Work out the finished part from the listing and answer in its coordinate system (mm). Face numbers are marked on the shaded views. A direction names the side the tool comes from. Give positions to 0.01 mm unless a question says otherwise; leave off trailing zeros. Write each loop counter-clockwise with the first axis right and the second up, starting at its lowest first coordinate (ties: lowest second). Pieces come first, ordered by that corner, then holes.
1) Determine the mould class of the marked faces 1, 2 and 3 for opening direction Z: pulls with the +Z half, pulls with the -Z half, needs draft (parallel to the pull), parting line crosses it, or undercut.
2) Straight lines are drawn through the part: probe 1 along X at (y, z) = (2.35, -15.5); probe 2 along X at (y, z) = (0.75, -1). For each, find the intervals that lie inside material, in ascending order.
3) Find section B-B (y = 3.4). Count the separate pieces of the cut face and the enclosed holes in it, plus the area to 3 significant figures.
4) Given pin 1 Ø3 at (x, z) = (9, 21) entering from +Y; pin 2 Ø4 at (x, z) = (10.5, 16) entering from +Y, each flat-ended and moving along its own axis, determine where each tip first touches the part or whether it passes through.
5) Find section A-A (z = 26). Determine the outline of the cut face in (x, y).
6) A tool of negligible diameter and unlimited length cuts with its end or side. For the marked faces 4 and 5, from which of +Z, -Z, +X, -X, +Y, -Y can it reach the whole face along a straight path? Write none if from no direction.
Autodesk Fusion 360 part; units mm, degrees
sketch "Sketch1" plane through (0, 0, 0) normal (0, 1, 0) x (1, 0, 0)
  line L0 (35, 35) -> (-35, 35)
  line L1 (-35, 35) -> (-35, -35)
  line L2 (-35, -35) -> (35, -35)
  line L3 (35, -35) -> (35, 35)
  line L4 (35, 35) -> (-35, -35) construction
  line L5 (-35, 35) -> (35, -35) construction
  line L6 (0, 0) -> (9.2688, 9.2688) construction
  line L7 (0, 0) -> (84.8528, 84.8528) construction
  line L8 (0, 0) -> (0, 35) construction
  line L9 (12.5, 35) -> (-12.5, 35)
  line L10 (-35, 12.5) -> (-35, -12.5)
  line L11 (-12.5, -35) -> (12.5, -35)
  line L12 (35, -12.5) -> (35, 12.5)
  line L13 (20.5061, 33.234) -> (33.234, 20.5061) construction
  line L14 (23.3345, 36.0624) -> (36.0624, 23.3345)
  line L15 (12.5, 35) -> (23.3345, 36.0624)
  line L16 (35, 12.5) -> (36.0624, 23.3345)
  circle A0 centre (22.6274, 31.1127) radius 1.6
  circle A1 centre (31.1127, 22.6274) radius 1.6
  line L17 (-35, 12.5) -> (-36.0624, 23.3345)
  line L18 (-36.0624, 23.3345) -> (-23.3345, 36.0624)
  line L19 (-12.5, 35) -> (-23.3345, 36.0624)
  circle A2 centre (-22.6274, 31.1127) radius 1.6
  circle A3 centre (-31.1127, 22.6274) radius 1.6
  line L20 (-12.5, -35) -> (-23.3345, -36.0624)
  line L21 (-23.3345, -36.0624) -> (-36.0624, -23.3345)
  line L22 (-35, -12.5) -> (-36.0624, -23.3345)
  circle A4 centre (-31.1127, -22.6274) radius 1.6
  circle A5 centre (-22.6274, -31.1127) radius 1.6
  line L23 (35, -12.5) -> (36.0624, -23.3345)
  line L24 (36.0624, -23.3345) -> (23.3345, -36.0624)
  line L25 (12.5, -35) -> (23.3345, -36.0624)
  circle A6 centre (22.6274, -31.1127) radius 1.6
  circle A7 centre (31.1127, -22.6274) radius 1.6
  dimension "d3" = 70
  dimension "d4" = 70
  dimension "d5" = 120
  dimension "d6" = 25
  dimension "d7" = 12.5
  dimension "d9" = 360
  dimension "d12" = 82
  dimension "d13" = 9
  dimension "d15" = 4
  dimension "d16" = 3.2
  dimension "d17" = 6
  dimension "d18" = 6
  dimension "d20" = 360
extrude "Extrude1" add sketch "Sketch1" along normal blind 4 contours L0 L1 L2 L3 L9 L10 L11 L12 L14 L18 L21 L24
sketch "Sketch2" plane through (0, 4, 0) normal (0, 1, 0) x (-1, 0, 0)
  circle A0 centre (-22.6274, 31.1127) radius 1.6
  circle A1 centre (-31.1127, 22.6274) radius 1.6
  circle A2 centre (31.1127, -22.6274) radius 1.6
  circle A3 centre (31.1127, 22.6274) radius 1.6
  circle A4 centre (22.6274, 31.1127) radius 1.6
  circle A5 centre (22.6274, -31.1127) radius 1.6
  circle A6 centre (-31.1127, -22.6274) radius 1.6
  circle A7 centre (-22.6274, -31.1127) radius 1.6
  line L0 (24.397, 35) -> (-24.397, 35)
  line L1 (-24.397, 35) -> (-35, 24.397)
  line L2 (-35, 24.397) -> (-35, -24.397)
  line L3 (-35, -24.397) -> (-24.397, -35)
  line L4 (-24.397, -35) -> (24.397, -35)
  line L5 (24.397, -35) -> (35, -24.397)
  line L6 (35, -24.397) -> (35, 24.397)
  line L7 (35, 24.397) -> (24.397, 35)
  line L8 (0, 0) -> (0, -35) construction
  line L9 (0, 0) -> (35, 0) construction
  line L10 (17.669, -29) -> (-17.669, -29)
  line L11 (-17.669, -29) -> (-29, -17.669)
  line L12 (-29, -17.669) -> (-29, 17.669)
  line L13 (-29, 17.669) -> (-17.669, 29)
  line L14 (-17.669, 29) -> (17.669, 29)
  line L15 (17.669, 29) -> (29, 17.669)
  line L16 (29, 17.669) -> (29, -17.669)
  line L17 (29, -17.669) -> (17.669, -29)
  dimension "d23" = 6
  dimension "d24" = 6
  dimension "d25" = 9
  dimension "d26" = 9
extrude "Extrude2" cut sketch "Sketch2" against normal blind 2 contours L10 L11 L12 L13 L14 L15 L16 L17
sketch "Sketch3" plane through (0, 2, 0) normal (0, 1, 0) x (-1, 0, 0)
  line L0 (29, -17.669) -> (29, 17.669)
  line L1 (29, 17.669) -> (17.669, 29)
  line L2 (17.669, 29) -> (-17.669, 29)
  line L3 (-17.669, 29) -> (-29, 17.669)
  line L4 (-29, 17.669) -> (-29, -17.669)
  line L5 (-29, -17.669) -> (-17.669, -29)
  line L6 (-17.669, -29) -> (17.669, -29)
  line L7 (17.669, -29) -> (29, -17.669)
  line L8 (0, 0) -> (0, -29) construction
  line L9 (0, 0) -> (29, 0) construction
  line L10 (15, -3.7839) -> (15, 4.5951)
  line L11 (16.0792, 6.8995) -> (24.0792, 13.5676)
  line L12 (15, -6) -> (15.0349, -6)
  line L13 (17.0557, -6.7828) -> (23.9792, -13.0929)
  line L14 (29, -10.8757) -> (29, 11.2631)
  arc A0 (23.9792, -13.0929) -> (29, -10.8757) centre (26, -10.8757) ccw
  arc A1 (29, 11.2631) -> (24.0792, 13.5676) centre (26, 11.2631) ccw
  arc A2 (16.0792, 6.8995) -> (15, 4.5951) centre (18, 4.5951) ccw
  arc A3 (17.0557, -6.7828) -> (16.5174, -6.3919) centre (15.0349, -9) ccw
  arc A4 (15, -3.7839) -> (16.5174, -6.3919) centre (18, -3.7839) ccw
  arc A5 (13.0929, 23.9792) -> (10.8757, 29) centre (10.8757, 26) ccw
  line L15 (10.8757, 29) -> (-11.2631, 29)
  line L16 (6.7828, 17.0557) -> (13.0929, 23.9792)
  arc A6 (-11.2631, 29) -> (-13.5676, 24.0792) centre (-11.2631, 26) ccw
  line L17 (-6.8995, 16.0792) -> (-13.5676, 24.0792)
  arc A7 (-6.8995, 16.0792) -> (-4.5951, 15) centre (-4.5951, 18) ccw
  line L18 (3.7839, 15) -> (-4.5951, 15)
  arc A8 (3.7839, 15) -> (6.3919, 16.5174) centre (3.7839, 18) ccw
  arc A9 (-23.9792, 13.0929) -> (-29, 10.8757) centre (-26, 10.8757) ccw
  line L19 (-29, 10.8757) -> (-29, -11.2631)
  line L20 (-17.0557, 6.7828) -> (-23.9792, 13.0929)
  arc A10 (-29, -11.2631) -> (-24.0792, -13.5676) centre (-26, -11.2631) ccw
  line L21 (-16.0792, -6.8995) -> (-24.0792, -13.5676)
  arc A11 (-16.0792, -6.8995) -> (-15, -4.5951) centre (-18, -4.5951) ccw
  line L22 (-15, 3.7839) -> (-15, -4.5951)
  arc A12 (-15, 3.7839) -> (-16.5174, 6.3919) centre (-18, 3.7839) ccw
  arc A13 (-13.0929, -23.9792) -> (-10.8757, -29) centre (-10.8757, -26) ccw
  line L23 (-10.8757, -29) -> (11.2631, -29)
  line L24 (-6.7828, -17.0557) -> (-13.0929, -23.9792)
  arc A14 (11.2631, -29) -> (13.5676, -24.0792) centre (11.2631, -26) ccw
  line L25 (6.8995, -16.0792) -> (13.5676, -24.0792)
  arc A15 (6.8995, -16.0792) -> (4.5951, -15) centre (4.5951, -18) ccw
  line L26 (-3.7839, -15) -> (4.5951, -15)
  arc A16 (-3.7839, -15) -> (-6.3919, -16.5174) centre (-3.7839, -18) ccw
  line L27 (10.8757, 29) -> (-11.2631, 29)
  point P0 (15, 6)
  dimension "d29" = 15
  dimension "d30" = 12
  dimension "d31" = 6
  dimension "d32" = 3
  dimension "d34" = 360
extrude "Extrude3" cut sketch "Sketch3" against normal blind 1.5 contours L0 L10 L11 L13 L14 A0 A1 A2 A3 A4
pattern_circular "C-Pattern1" count 4 over 360 about axis through (0, 1.75, 0) along (0, 1, 0) of "Extrude3"
sketch "Sketch4" plane through (0, 2, 0) normal (0, 1, 0) x (-1, 0, 0)
  arc A0 (-13.0929, -23.9792) -> (-10.8757, -29) centre (-10.8757, -26) ccw
  line L0 (-13.0929, -23.9792) -> (-6.7828, -17.0557)
  arc A1 (-6.7828, -17.0557) -> (-6.3919, -16.5174) centre (-9, -15.0349) ccw
  arc A2 (-3.7839, -15) -> (-6.3919, -16.5174) centre (-3.7839, -18) ccw
  line L1 (-3.7839, -15) -> (4.5951, -15)
  arc A3 (6.8995, -16.0792) -> (4.5951, -15) centre (4.5951, -18) ccw
  line L2 (6.8995, -16.0792) -> (13.5676, -24.0792)
  arc A4 (11.2631, -29) -> (13.5676, -24.0792) centre (11.2631, -26) ccw
  line L3 (11.2631, -29) -> (17.669, -29)
  line L4 (17.669, -29) -> (29, -17.669)
  line L5 (29, -17.669) -> (29, -10.8757)
  arc A5 (23.9792, -13.0929) -> (29, -10.8757) centre (26, -10.8757) ccw
  line L6 (23.9792, -13.0929) -> (17.0557, -6.7828)
  arc A6 (17.0557, -6.7828) -> (16.5174, -6.3919) centre (15.0349, -9) ccw
  arc A7 (15, -3.7839) -> (16.5174, -6.3919) centre (18, -3.7839) ccw
  line L7 (15, -3.7839) -> (15, 4.5951)
  arc A8 (16.0792, 6.8995) -> (15, 4.5951) centre (18, 4.5951) ccw
  line L8 (16.0792, 6.8995) -> (24.0792, 13.5676)
  arc A9 (29, 11.2631) -> (24.0792, 13.5676) centre (26, 11.2631) ccw
  line L9 (29, 11.2631) -> (29, 17.669)
  line L10 (29, 17.669) -> (17.669, 29)
  line L11 (17.669, 29) -> (10.8757, 29)
  arc A10 (13.0929, 23.9792) -> (10.8757, 29) centre (10.8757, 26) ccw
  line L12 (13.0929, 23.9792) -> (6.7828, 17.0557)
  arc A11 (6.7828, 17.0557) -> (6.3919, 16.5174) centre (9, 15.0349) ccw
  arc A12 (3.7839, 15) -> (6.3919, 16.5174) centre (3.7839, 18) ccw
  line L13 (3.7839, 15) -> (-4.5951, 15)
  arc A13 (-6.8995, 16.0792) -> (-4.5951, 15) centre (-4.5951, 18) ccw
  line L14 (-6.8995, 16.0792) -> (-13.5676, 24.0792)
  arc A14 (-11.2631, 29) -> (-13.5676, 24.0792) centre (-11.2631, 26) ccw
  line L15 (-11.2631, 29) -> (-17.669, 29)
  line L16 (-17.669, 29) -> (-29, 17.669)
  line L17 (-29, 17.669) -> (-29, 10.8757)
  arc A15 (-23.9792, 13.0929) -> (-29, 10.8757) centre (-26, 10.8757) ccw
  line L18 (-23.9792, 13.0929) -> (-17.0557, 6.7828)
  arc A16 (-17.0557, 6.7828) -> (-16.5174, 6.3919) centre (-15.0349, 9) ccw
  arc A17 (-15, 3.7839) -> (-16.5174, 6.3919) centre (-18, 3.7839) ccw
  line L19 (-15, 3.7839) -> (-15, -4.5951)
  arc A18 (-16.0792, -6.8995) -> (-15, -4.5951) centre (-18, -4.5951) ccw
  line L20 (-16.0792, -6.8995) -> (-24.0792, -13.5676)
  arc A19 (-29, -11.2631) -> (-24.0792, -13.5676) centre (-26, -11.2631) ccw
  line L21 (-29, -11.2631) -> (-29, -17.669)
  line L22 (-29, -17.669) -> (-17.669, -29)
  line L23 (-17.669, -29) -> (-10.8757, -29)
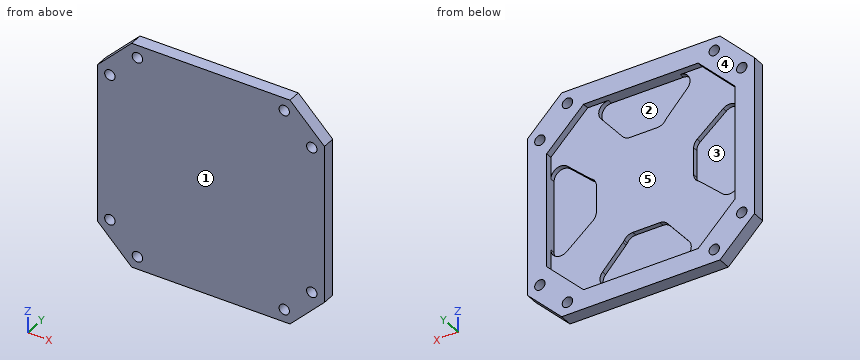
Results:
1. face 1: needs draft
1. face 2: undercut
1. face 3: undercut
2. probe 1: x = -35 to -29, 29 to 35
2. probe 2: x = -35 to -29, -15 to 15, 29 to 35
3. separate pieces: 1
3. enclosed holes: 9
3. area: 1,500 mm2
4. pin 1: stops at y = 0.5
4. pin 2: stops at y = 2
5. outline: (-33.4, 0) - (33.4, 0) - (33.4, 4) - (20.67, 4) - (20.67, 2) - (14.26, 2) - (14.26, 0.5) - (-13.88, 0.5) - (-13.88, 2) - (-20.67, 2) - (-20.67, 4) - (-33.4, 4) - close
6. face 4: +Z, -Z, +X, -X, +Y
6. face 5: +Y
